from build123d import *

# Parameters (mm, degrees)
F0_R     = 70
F0_W     = 18.4
F0_H     = 3.4
F0_W_2   = 64.3
F0_R_2   = 4.1
F1_DEPTH = 3.2
F2_R     = 1.65
F3_DEPTH = 3.2


with BuildPart() as f1:
    # F0 (on Top) → F1 (new body)
    with BuildSketch(Plane.XY):
        Circle(F0_R)
        with Locations((-54.2, -14.2)):
            Rectangle(F0_W, F0_H, mode=Mode.SUBTRACT)
        with Locations((-2.85, -26.7)):
            Rectangle(F0_W_2, F0_H, mode=Mode.SUBTRACT)
        with Locations((-54.2, 14.2)):
            Rectangle(F0_W, F0_H, mode=Mode.SUBTRACT)
        with Locations((-2.85, 26.7)):
            Rectangle(F0_W_2, F0_H, mode=Mode.SUBTRACT)
        Circle(F0_R_2, mode=Mode.SUBTRACT)
    extrude(amount=-F1_DEPTH)

    # F2 (on Top) → F3 (cut)
    with BuildSketch(Plane.XY):
        with Locations((14.707094, -55.149738)):
            Circle(F2_R)
    extrude(amount=-F3_DEPTH, mode=Mode.SUBTRACT)


solid = f1.part
Design review of the part built by this model. Coordinates are the model's own, in mm. Give positions to 0.01 mm unless a question says otherwise; leave off trailing zeros. Loops run counter-clockwise (first coordinate to the right, second up) from the corner with the lowest first, then second, coordinate; pieces in that order, holes last. Notation, with made-up numbers: (63, 44) - (73, 44) arc R19 cw to (73, 59) - close; hole circle Ø10 at (-14.75, 23). An arc over 180 degrees is marked (long way). Use CSV: the item, a comma, the result in double quotes. Start each with the question number.
1. Wall thickness on L1, parallel to Y at x = 0, z = -1.05; L2, parallel to Y at x = -11, z = -1.75; L3, parallel to Y at x = -57, z = -1.3: over which ranges is each line inside the solid? List them lowest first.
2. Insertion check: P1, Ø1, axis at y = -15, z = -1, coming from the +X side; P2, Ø1.6, axis at y = 26, z = -1, coming from the -X side; P3, Ø1, axis at y = -47.5, z = -2.5, coming from the -X side. Each pin has a flat end and moves straight along its axis. Give the tip position at first contact, or say it passes through.
3. Draft analysis for pull direction Y (two halves, no side actions). For faces 1 (the flat face through (15, 1, -3.2)), 2 (the flat face through (-3, 25, -2)), 3 (the cylindrical face through (-55.55, -42.594, -1.578)), state which applies: released by +Y, released by -Y, zero draft, split by the parting line, or undercut.
4. Add section A-A (x = 0). State the section outline as (y, z) points.
5. Add section C-C (x = -16). State the section outline as (y, z) points.
6. Add section D-D (z = -2.7). State the section outline as (x, y) points.
7. Add section B-B (y = 0). State the section outline as (x, z) points, plus the area to 3 significant figures.
Results found:
1,L1,"y = -70 to -28.4, -25 to -4.1, 4.1 to 25, 28.4 to 70"
1,L2,"y = -69.13 to -28.4, -25 to 25, 28.4 to 69.13"
1,L3,"y = -40.63 to -15.9, -12.5 to 12.5, 15.9 to 40.63"
2,P1,"stops at x = 68.48"
2,P2,"stops at x = -65.31"
2,P3,"stops at x = -51.87"
3,face 1,"zero draft"
3,face 2,"undercut"
3,face 3,"split by the parting line"
4,outline,"(-70, -3.2) - (-28.4, -3.2) - (-28.4, 0) - (-70, 0) - close; (-25, -3.2) - (-4.1, -3.2) - (-4.1, 0) - (-25, 0) - close; (4.1, -3.2) - (25, -3.2) - (25, 0) - (4.1, 0) - close; (28.4, -3.2) - (70, -3.2) - (70, 0) - (28.4, 0) - close"
5,outline,"(-68.15, -3.2) - (-28.4, -3.2) - (-28.4, 0) - (-68.15, 0) - close; (-25, -3.2) - (25, -3.2) - (25, 0) - (-25, 0) - close; (28.4, -3.2) - (68.15, -3.2) - (68.15, 0) - (28.4, 0) - close"
6,outline,"circle Ø140 at (0, 0); hole (-63.4, -15.9) - (-45, -15.9) - (-45, -12.5) - (-63.4, -12.5) - close; hole (-63.4, 12.5) - (-45, 12.5) - (-45, 15.9) - (-63.4, 15.9) - close; hole (-35, -28.4) - (29.3, -28.4) - (29.3, -25) - (-35, -25) - close; hole (-35, 25) - (29.3, 25) - (29.3, 28.4) - (-35, 28.4) - close; hole circle Ø8.2 at (0, 0); hole circle Ø3.3 at (14.71, -55.15)"
7,outline,"(-70, -3.2) - (-4.1, -3.2) - (-4.1, 0) - (-70, 0) - close; (4.1, -3.2) - (70, -3.2) - (70, 0) - (4.1, 0) - close"
7,area,"422 mm²"
